Source: CAD feature listing. Evaluate the final solid. Frame: model axes, mm. A direction names the side the tool comes from. Round coordinates to 2 decimals unless told otherwise and drop trailing zeros. Order: outer loops, then holes, each group sorted by start corner. A loop starts at its lowest first (then second) coordinate and runs counter-clockwise, first axis right, second up. Notation, with made-up numbers: (6.5, 50.5) - (60.5, 50.5) arc R21 cw to (60.5, 83.5) - close; hole circle Ø9 at (-30, 46.5). An arc over 180 degrees is marked (long way). Return JSON: item names as keys, results as strings. Group by question number.
1) Section C-C, the plane z = 28.5. Return loops of the section in (x, y).
2) Ray query, line 1 (Z direction, x = 0, y = 4.75); line 2 (Y direction, x = 0, z = 6); line 3 (Z direction, x = 0, y = 0.75). Return the intervals inside material, ascending. Write a range as from..to.
3) Contact query for flat-ended pins moving along their axis: P1, Ø7, axis at x = 0, y = 0, coming from the -Z side; P2, Ø6, axis at x = -2.5, z = 32, coming from the +Y side; P3, Ø1, axis at x = -7.5, y = -1, coming from the +Z side. Output: stop coordinate, or through.
4) Access query for faces 4 (the flat face through (-0.1, -5, 37.4)), 5 (the flat face through (0, 5, 10)), 6 (the flat face through (0, 0, 25)). Directions: +Z, -Z, +X, -X, +Y, -Y. A direction counts if a zero-diameter tool reaches every point of the face in a straight line with its end or side. Return the directions, or none.
5) Section A-A, the plane y = 0. Return loops of the section in (x, z), plus the area to 3 significant figures.
6) Section B-B, the plane x = 0. Give the number of separate pieces and of enclosed holes in the cut face, plus the area to 3 significant figures.
7) Mould query, pull axis Z, two halves, no side actions, for faces 1 (the flat face through (0, -7, 13)), 2 (the flat face through (0, 7, 23)), 3 (the flat face through (-0.1, 5, 37.4)). Classes: pulls with the +Z half, pulls with the -Z half, needs draft (parallel to the pull), parting line crosses it, or undercut.
```python
from build123d import *

# Parameters (mm, degrees)
F0_W      = 20
F0_H      = 20
F0_R      = 4
F1_DEPTH  = 25
F3_W      = 14
F3_H      = 5.8359876275
F4_DEPTH  = 17
F6_W      = 20
F6_H      = 10
F7_DEPTH  = 15
F10_DEPTH = 10
F9_R      = 5.5
F11_DEPTH = 10
F12_SIZE  = 4.99999


# Not quite as in the source:
# - a fillet or chamfer is up to 0.001 mm smaller than in the source, because OpenCascade refuses the exact size


with BuildPart() as f1:
    # F0 (on Top) → F1 (new body)
    with BuildSketch(Plane.XY):
        Rectangle(F0_W, F0_H)
        Circle(F0_R, mode=Mode.SUBTRACT)
    extrude(amount=F1_DEPTH)

    # F3 (on offset) → F4 (cut)
    with BuildSketch(Plane(origin=(0, 10, 0), x_dir=(-1, 0, 0), z_dir=(0, 1, 0))):
        with Locations((0, 12.9179938138)):
            Rectangle(F3_W, F3_H)
    extrude(amount=-F4_DEPTH, mode=Mode.SUBTRACT)

    # F6 (on offset) → F7 (join)
    with BuildSketch(Plane.XY.offset(25)):
        Rectangle(F6_W, F6_H)
    extrude(amount=F7_DEPTH)

    # F9 (on offset) → F10 (cut)
    with BuildSketch(Plane(origin=(0, 5, 0), x_dir=(-1, 0, 0), z_dir=(0, 1, 0))):
        with BuildLine():
            Line((-5.2678268764, 40), (-10, 40))
            Line((-10, 40), (-10, 31.5))
            ThreePointArc((-10, 31.5), (-8.7372269275, 36.3642435813), (-5.2678268764, 40))
        make_face()
        with BuildLine():
            Line((10, 40), (5.2678268764, 40))
            ThreePointArc((5.2678268764, 40), (8.7372269275, 36.3642435813), (10, 31.5))
            Line((10, 31.5), (10, 40))
        make_face()
    extrude(amount=-F10_DEPTH, mode=Mode.SUBTRACT)

    # F9 (on offset) → F11 (cut)
    with BuildSketch(Plane(origin=(0, 5, 0), x_dir=(-1, 0, 0), z_dir=(0, 1, 0))):
        with Locations((0, 31.5)):
            Circle(F9_R)
    extrude(amount=-F11_DEPTH, mode=Mode.SUBTRACT)

    # F12 (size 5 in the source; OpenCascade refuses exactly that, so slightly less here)
    f12_edges = [f1.edges().sort_by_distance(p)[0] for p in [
        (0, -10, 25),
        (0, 10, 25),
    ]]
    chamfer(f12_edges, length=F12_SIZE)


solid = f1.part
```
Geometry check:
{
 "1": {"outline": "(-10, -5) - (-4.61, -5) - (-4.61, 5) - (-10, 5) - close; (4.61, -5) - (10, -5) - (10, 5) - (4.61, 5) - close"},
 "2": {"line 1": "0..10, 15.84..26, 37..40", "line 2": "-10..-4, 4..10", "line 3": "25..26, 37..40"},
 "3": {"P1": "z = 25", "P2": "y = 5", "P3": "z = 38.64"},
 "4": {"face 4": "+Z, +X, -X, -Y", "face 5": "+Y", "face 6": "-Z"},
 "5": {"outline": "(-10, 0) - (-4, 0) - (-4, 10) - (-7, 10) - (-7, 15.84) - (-4, 15.84) - (-4, 25) - (4, 25) - (4, 15.84) - (7, 15.84) - (7, 10) - (4, 10) - (4, 0) - (10, 0) - (10, 31.5) arc R10 ccw to (5.27, 40) - (-5.27, 40) arc R10 ccw to (-10, 31.5) - close; hole circle Ø11 at (0, 31.5)", "area": "446 mm2"},
 "6": {"separate pieces": "3", "enclosed holes": "0", "area": "262 mm2"},
 "7": {"face 1": "undercut", "face 2": "pulls with the +Z half", "face 3": "needs draft"}
}
